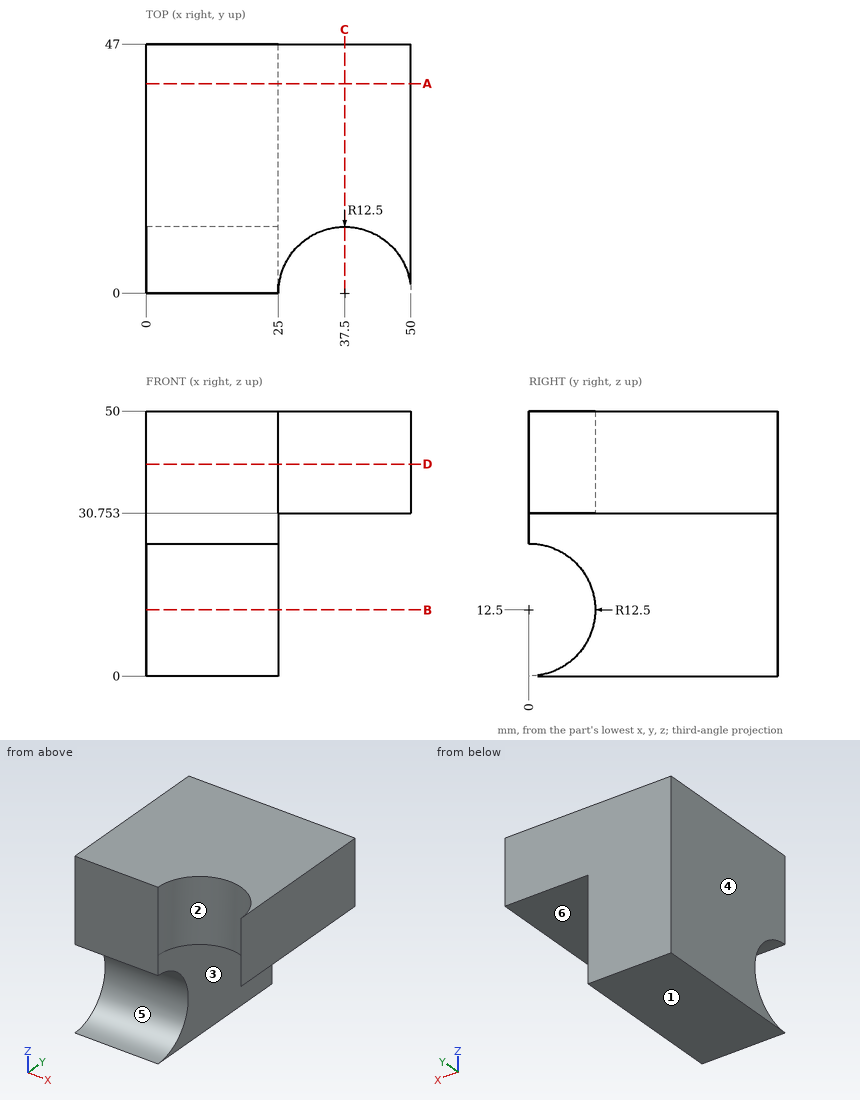
Answer from the drawing. Dimensions are ordinates in mm from the lowest x, y and z of the part. A direction names the side the tool comes from. Round coordinates to 2 decimals unless told otherwise and drop trailing zeros. Write each loop counter-clockwise with the first axis right and the second up, starting at its lowest first coordinate (ties: lowest second). Pieces come first, ordered by that corner, then holes.
1. Which of the six approach directions +Z, -Z, +X, -X, +Y, -Y give full straight-line access (tool end or side, diameter ignored) to the marked faces 5 and 6?
2. The part is cut by section B-B, the plane z = 12.5. Determine the outline of the cut face in (x, y).
3. Straight lines are drawn through the part: L1, parallel to X at y = 42.5, z = 30.5; L2, parallel to Y at x = 38, z = 31; L3, parallel to Z at x = 14, y = 3. For each, find the intervals that lie inside material, in ascending order.
4. Determine the mould class of the marked faces 1, 2, 3 and 4 for opening direction X: pulls with the +X half, pulls with the -X half, needs draft (parallel to the pull), parting line crosses it, or undercut.
5. The part is cut by section A-A, the plane y = 39.5. Determine the outline of the cut face in (x, z), then the cut area to 3 significant figures.
6. The part is cut by section D-D, the plane z = 40. Determine the outline of the cut face in (x, y), then the cut area to 3 significant figures.
7. The part is cut by section C-C, the plane x = 37.5. Determine the outline of the cut face in (y, z), then the cut area to 3 significant figures.
8. Given pin 1 Ø15.5 at (y, z) = (25, 19.5) entering from +X, flat-ended and moving along its own axis, determine where the tip first touches the part or whether it passes through.
Values:
1. face 5: +X, -X, -Y
1. face 6: -Z, +X, +Y, -Y
2. outline: (0, 12.5) - (25, 12.5) - (25, 47) - (0, 47) - close
3. L1: x = 0 to 25
3. L2: y = 12.49 to 47
3. L3: z = 0 to 0.37, 24.63 to 50
4. face 1: needs draft
4. face 2: undercut
4. face 3: pulls with the +X half
4. face 4: pulls with the -X half
5. outline: (0, 0) - (25, 0) - (25, 30.75) - (50, 30.75) - (50, 50) - (0, 50) - close
5. area: 1,730 mm2
6. outline: (0, 0) - (25, 0) arc R12.5 cw to (50, 0) - (50, 47) - (0, 47) - close
6. area: 2,100 mm2
7. outline: (12.5, 30.75) - (47, 30.75) - (47, 50) - (12.5, 50) - close
7. area: 664 mm2
8. pin 1: stops at x = 25
